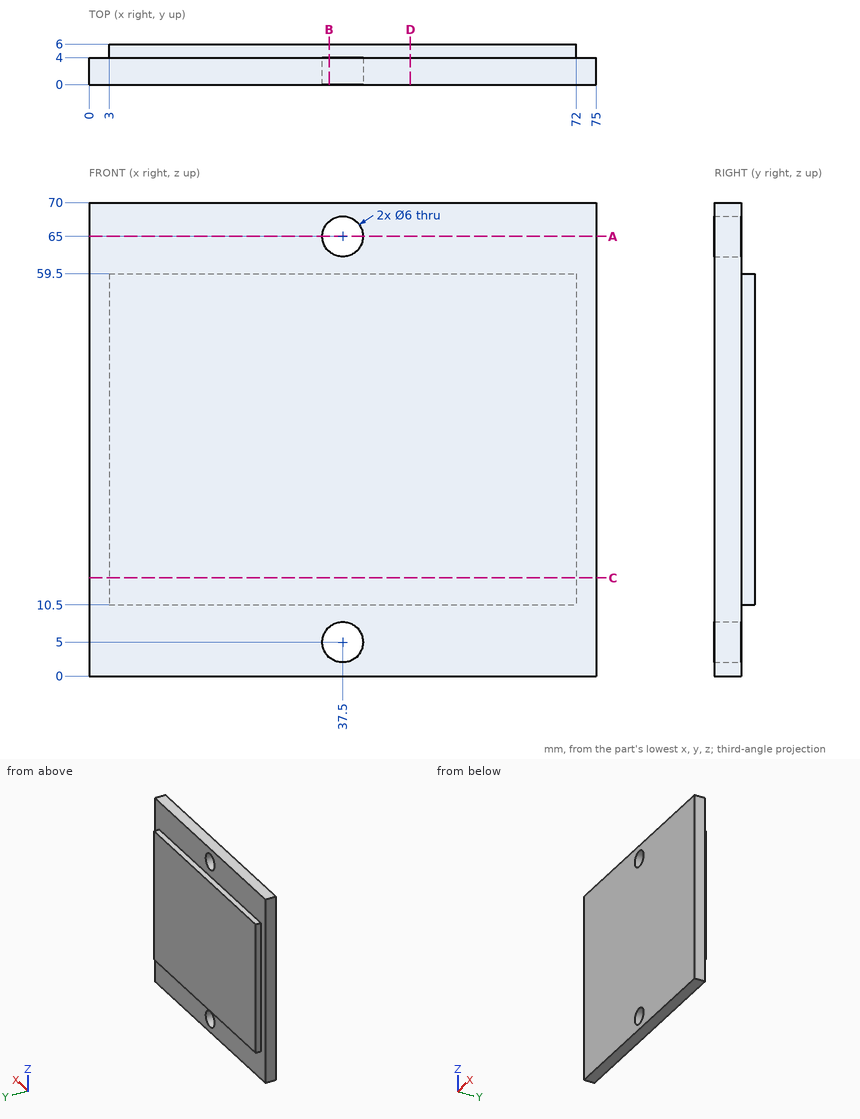
Job drawing, mm, ordinate dimensions from the low corner. One solid piece. Round coordinates to 2 decimals unless told otherwise and drop trailing zeros. Loops run counter-clockwise (first coordinate to the right, second up) from the corner with the lowest first, then second, coordinate; pieces in that order, holes last. Notation, with made-up numbers: (-14.5, 14) -> (43.5, 14) arc R14 ccw to (43.5, 21) -> close; hole circle Ø7 at (87, 28.25). An arc over 180 degrees is marked (long way). Use a Markdown table: item, result.
1) Probe line 1 (Z direction, x = 37.5, y = 1); line 2 (Z direction, x = 41, y = 5.2); line 3 (X direction, y = 0.85, z = 65). List the from-to ranges inside material, lowest first. Write a range as [from, to].
The answers:
| item | result |
|---|---|
| line 1 | z = [0, 2], [8, 62], [68, 70] |
| line 2 | z = [10.5, 59.5] |
| line 3 | x = [0, 34.5], [40.5, 75] |
2) Drop flat-ended pins along their axis: pin 1 Ø9.5 at (x, z) = (37.5, 5) entering from +Y; pin 2 Ø1 at (x, y) = (31.5, 5) entering from -Z; pin 3 Ø1 at (y, z) = (5.5, 32) entering from -X. Give the stop position or say it passes through.
The answers:
| item | result |
|---|---|
| pin 1 | stops at y = 4 |
| pin 2 | stops at z = 10.5 |
| pin 3 | stops at x = 3 |
3) Cut at C-C, the plane z = 14.5. List the corners of the cut face in (x, y).
The answers:
| item | result |
|---|---|
| outline | (0, 0) -> (75, 0) -> (75, 4) -> (72, 4) -> (72, 6) -> (3, 6) -> (3, 4) -> (0, 4) -> close |
4) Cut at D-D, the plane x = 47.5. List the corners of the cut face in (y, z), and give its area (3 significant figures).
The answers:
| item | result |
|---|---|
| outline | (0, 0) -> (4, 0) -> (4, 10.5) -> (6, 10.5) -> (6, 59.5) -> (4, 59.5) -> (4, 70) -> (0, 70) -> close |
| area | 378 mm2 |
5) Cut at B-B, the plane x = 35.5. List the corners of the cut face in (y, z), and give its area (3 significant figures).
The answers:
| item | result |
|---|---|
| outline | (0, 0) -> (4, 0) -> (4, 2.76) -> (0, 2.76) -> close; (0, 7.24) -> (4, 7.24) -> (4, 10.5) -> (6, 10.5) -> (6, 59.5) -> (4, 59.5) -> (4, 62.76) -> (0, 62.76) -> close; (0, 67.24) -> (4, 67.24) -> (4, 70) -> (0, 70) -> close |
| area | 342 mm2 |
6) Cut at A-A, the plane z = 65. List the corners of the cut face in (x, y), and give its area (3 significant figures).
The answers:
| item | result |
|---|---|
| outline | (0, 0) -> (34.5, 0) -> (34.5, 4) -> (0, 4) -> close; (40.5, 0) -> (75, 0) -> (75, 4) -> (40.5, 4) -> close |
| area | 276 mm2 |
